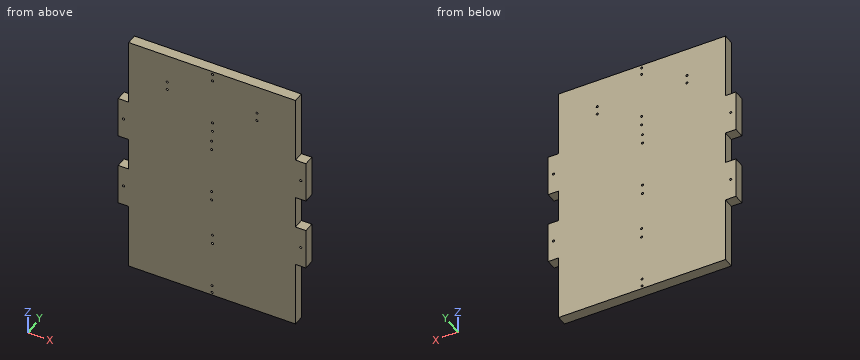
from build123d import *

# Parameters (mm, degrees)
SKETCH1_W           = 101.6
SKETCH1_H           = 152.4
BOSS_EXTRUDE1_DEPTH = 6.35
SKETCH2_W           = 25.498289586
SKETCH2_H           = 6.35
BOSS_EXTRUDE2_DEPTH = 6.35
SKETCH3_W           = 25.498289586
SKETCH3_H           = 6.35
BOSS_EXTRUDE3_DEPTH = 6.35
SKETCH4_R           = 0.635
CUT_EXTRUDE1_DEPTH  = 6.35
SKETCH5_R           = 0.635
CUT_EXTRUDE2_DEPTH  = 7.35
SKETCH7_R           = 0.635
CUT_EXTRUDE3_DEPTH  = 7.35
SKETCH9_R           = 0.635
CUT_EXTRUDE4_DEPTH  = 7.35


with BuildPart() as part:
    # Sketch1 → Boss-Extrude1 (new body)
    with BuildSketch(Plane(origin=(0, 0, 0), x_dir=(1, 0, 0), z_dir=(0, 1, 0))):
        with Locations((50.8, 76.2)):
            Rectangle(SKETCH1_W, SKETCH1_H)
    extrude(amount=BOSS_EXTRUDE1_DEPTH)

    # Sketch2 → Boss-Extrude2 (add)
    with BuildSketch(Plane(origin=(101.6, 0, 0), x_dir=(0, 0, -1), z_dir=(1, 0, 0))):
        with Locations((53.389144793, 3.175)):
            Rectangle(SKETCH2_W, SKETCH2_H)
        with Locations((99.010855207, 3.175)):
            Rectangle(SKETCH2_W, SKETCH2_H)
    extrude(amount=BOSS_EXTRUDE2_DEPTH)

    # Sketch3 → Boss-Extrude3 (add)
    with BuildSketch(Plane.ZY):
        with Locations((-99.010855207, 3.175)):
            Rectangle(SKETCH3_W, SKETCH3_H)
        with Locations((-53.389144793, 3.175)):
            Rectangle(SKETCH3_W, SKETCH3_H)
    extrude(amount=BOSS_EXTRUDE3_DEPTH)

    # Sketch4 → Cut-Extrude1 (cut)
    with BuildSketch(Plane.XZ):
        with Locations((-3.175, -53.389144793)):
            Circle(SKETCH4_R)
        with Locations((-3.175, -99.010855207)):
            Circle(SKETCH4_R)
        with Locations((104.775, -53.389144793)):
            Circle(SKETCH4_R)
        with Locations((104.775, -99.010855207)):
            Circle(SKETCH4_R)
    extrude(amount=-CUT_EXTRUDE1_DEPTH, mode=Mode.SUBTRACT)

    # Sketch5 → Cut-Extrude2 (cut, through all)
    with BuildSketch(Plane.XZ):
        with Locations((51.054, -6.304558397)):
            Circle(SKETCH5_R)
        with Locations((51.054001096, -34.940813016)):
            Circle(SKETCH5_R)
        with Locations((51.054, -40.655813016)):
            Circle(SKETCH5_R)
        with Locations((51.054, -1.859558397)):
            Circle(SKETCH5_R)
        with Locations((50.530750765, -87.704154674)):
            Circle(SKETCH5_R)
        with Locations((50.546, -47.628968946)):
            Circle(SKETCH5_R)
        with Locations((50.546, -53.343968946)):
            Circle(SKETCH5_R)
        with Locations((50.544258636, -81.989170638)):
            Circle(SKETCH5_R)
        with Locations((51.054, -111.498317742)):
            Circle(SKETCH5_R)
        with Locations((51.054, -117.213317742)):
            Circle(SKETCH5_R)
    extrude(amount=-CUT_EXTRUDE2_DEPTH, mode=Mode.SUBTRACT)

    # Sketch7 → Cut-Extrude3 (cut, through all)
    with BuildSketch(Plane(origin=(0, 6.35, 0), x_dir=(1, 0, 0), z_dir=(0, 1, 0))):
        with Locations((23.495, 17.78)):
            Circle(SKETCH7_R)
        with Locations((23.495, 22.86)):
            Circle(SKETCH7_R)
        with Locations((78.105, 22.86)):
            Circle(SKETCH7_R)
        with Locations((78.105, 17.78)):
            Circle(SKETCH7_R)
    extrude(amount=-CUT_EXTRUDE3_DEPTH, mode=Mode.SUBTRACT)

    # Sketch9 → Cut-Extrude4 (cut, through all)
    with BuildSketch(Plane(origin=(0, 6.35, 0), x_dir=(1, 0, 0), z_dir=(0, 1, 0))):
        with Locations((50.8, 150.622)):
            Circle(SKETCH9_R)
        with Locations((50.8, 146.05)):
            Circle(SKETCH9_R)
    extrude(amount=-CUT_EXTRUDE4_DEPTH, mode=Mode.SUBTRACT)


solid = part.part
Read the model definition and answer for the solid it produces. Units are mm, in the model's axes. Round coordinates to 2 decimals unless told otherwise and drop trailing zeros. Loops run counter-clockwise (first coordinate to the right, second up) from the corner with the lowest first, then second, coordinate; pieces in that order, holes last. Notation, with made-up numbers: (-7, 14) - (45, 14) arc R30 cw to (45, 51) - close; hole circle Ø7 at (49, 59.5). An arc over 180 degrees is marked (long way). One line per question, with ' | ' between items. Start each with the question number.
Q1. Section A-A on z = -26.5 is taken. Give the vertices of the cut face in (x, y), plus the area to 3 significant figures.
Q2. Flat-ended cylindrical pins translate along their axes: pin 1 (1.5 mm diameter, centred on x = 51.05, z = -40.66, fed in from +Y); pin 2 (3 mm diameter, centred on y = 4.5, z = -25, fed in from +X); pin 3 (3 mm diameter, centred on y = 3, z = -24.5, fed in from -X); pin 4 (1.9 mm diameter, centred on x = -4.5, y = 3.5, fed in from -Z). Find the tip coordinate at first contact, or state that the pin passes through.
Q3. Find the intervals of material crossed by L1, parallel to X at y = 1.5, z = -17.78; L2, parallel to X at y = 3.5, z = -117; L3, parallel to X at y = 4, z = -21, in increasing order.
Q4. Section B-B on y = 3.25 is taken. Count the separate pieces of the cut face and the enclosed holes in it, plus the area to 3 significant figures.
Established:
1) outline: (0, 0) - (101.6, 0) - (101.6, 6.35) - (0, 6.35) - close | area: 645 mm²
2) pin 1: y = 6.35 | pin 2: x = 101.6 | pin 3: x = 0 | pin 4: z = -111.76
3) L1: 0 to 22.86, 24.13 to 77.47, 78.74 to 101.6 | L2: 0 to 50.46, 51.65 to 101.6 | L3: 0 to 101.6
4) separate pieces: 1 | enclosed holes: 20 | area: 16,100 mm²
